The model under review builds one solid part; all positions refer to its coordinate system, in mm. A direction names the side the tool comes from. Coordinates: 2 decimals unless noted, no trailing zeros. Order: outer loops, then holes, each group sorted by start corner. A loop starts at its lowest first (then second) coordinate and runs counter-clockwise, first axis right, second up. Notation, with made-up numbers: M 35.5,67 L 50.5,67 A26 cw 50.5,91 Z; hole C 17.25,62.5 d10. An arc over 180 degrees is marked long. Answer in a Markdown table with one row per item.
from build123d import *

# Parameters (mm, degrees)
SKETCH_5_R                   = 50
EXTRUDE_1_DEPTH              = 35
SKETCH_2_W                   = 22
SKETCH_2_H                   = 20
CUT_EXTRUDE_1_DEPTH          = 165.975755795
HOLE_WIZARD_M6_1_D           = 6.6
HOLE_WIZARD_M6_1_CBORE_D     = 11
HOLE_WIZARD_M6_1_CBORE_DEPTH = 6.4
CUT_EXTRUDE_START            = -15
CUT_EXTRUDE_5_DEPTH          = 15
SKETCH_7_R                   = 5


with BuildPart() as part:
    # 草圖1 → 旋轉1 (revolve)
    with BuildSketch(Plane(origin=(0, 0, 0), x_dir=(0, 0, -1), z_dir=(1, 0, 0))):
        Polygon((0, 0), (0, 20), (50, 20), (114, 10), (114, 0), align=None)
    revolve(axis=Axis((0, 0, 0), (0, 1, 0)))

    # 草圖5 → 填料-伸長1 (add)
    with BuildSketch(Plane(origin=(0, 20, 0), x_dir=(1, 0, 0), z_dir=(0, 1, 0))):
        with Locations(Location((0, 0, 0), (0, 0, 270))):
            Circle(SKETCH_5_R)
    extrude(amount=-EXTRUDE_1_DEPTH)

    # 草圖2 → 除料-伸長1 (cut, through all)
    with BuildSketch(Plane(origin=(0, 20, 0), x_dir=(1, 0, 0), z_dir=(0, 1, 0))):
        with Locations((0, 18)):
            Rectangle(SKETCH_2_W, SKETCH_2_H)
    extrude(amount=-CUT_EXTRUDE_1_DEPTH, mode=Mode.SUBTRACT)

    # M6 六角承窩頭蓋螺釘的柱孔1 (through all)
    with Locations(Plane(origin=(0, 20, 0), x_dir=(1, 0, 0), z_dir=(0, 1, 0))):
        with Locations((37.5, 11), (22.5, 11), (-22.5, 11), (-37.5, 11)):
            CounterBoreHole(HOLE_WIZARD_M6_1_D / 2, HOLE_WIZARD_M6_1_CBORE_D / 2, HOLE_WIZARD_M6_1_CBORE_DEPTH)

    # 草圖6 → 除料-伸長5 (cut)
    with BuildSketch(Plane.XZ.offset(15).offset(CUT_EXTRUDE_START)):
        with BuildLine():
            Line((-37.563279942, 33), (37.563279942, 33))
            ThreePointArc((37.563279942, 33), (0, 50), (-37.563279942, 33))
        make_face()
        with BuildLine():
            ThreePointArc((-37.563279942, -33), (0, -50), (37.563279942, -33))
            Line((37.563279942, -33), (-37.563279942, -33))
        make_face()
    extrude(amount=CUT_EXTRUDE_5_DEPTH, mode=Mode.SUBTRACT)

    # 掃出1: sweep along a path in 草圖8
    with BuildLine(Plane.XY.offset(8)) as sweep_1_path:
        ThreePointArc((37.792366216, 20), (0, 57.792366216), (-37.792366216, 20))
    # 草圖7 → 掃出1 (sweep)
    with BuildSketch(Plane(origin=(0, 20, 0), x_dir=(1, 0, 0), z_dir=(0, 1, 0))):
        with Locations((38, -8)):
            Circle(SKETCH_7_R)
    sweep(path=sweep_1_path.line)


solid = part.part
(1) Take a section at B-B (x = 0). Write out the cut boundary in (y, z), then the cut area to 3 significant figures.
Report:
| item | result |
|---|---|
| outline | M -15,-33 L 0,-33 L 0,-114 L 10,-114 L 20,-50 L 20,-28 L -15,-28 Z; M -15,-8 L 20,-8 L 20,50 L 10,114 L 0,114 L 0,33 L -15,33 Z; C 58,8 d10 |
| area | 4,290 mm^2 |
(2) Take a section at A-A (y = 16.5). Write out the cut boundary in (x, z), then the cut area to 3 significant figures.
Report:
| item | result |
|---|---|
| outline | C 0,0 d144.8; hole C -37.5,-11 d11; hole C -22.5,-11 d11; hole M -11,-28 L 11,-28 L 11,-8 L -11,-8 Z; hole C 22.5,-11 d11; hole C 37.5,-11 d11 |
| area | 15,600 mm^2 |
(3) Take a section at C-C (z = -11). State how many separate pieces and enclosed holes the cut face has, then the cut area to 3 significant figures.
Report:
| item | result |
|---|---|
| separate pieces | 6 |
| enclosed holes | 0 |
| area | 3,550 mm^2 |
(4) Insertion check: P1, Ø8, axis at y = 1, z = 57, coming from the -X side; P2, Ø1.5, axis at x = -38.5, z = 50.5, coming from the +Y side; P3, Ø12, axis at y = -2, z = -23, coming from the -X side. Each pin has a flat end and moves straight along its axis. Give the tip position at first contact, or say it passes through.
Report:
| item | result |
|---|---|
| P1 | x = -100.93 |
| P2 | y = 18.01 |
| P3 | x = -112.67 |
(5) The part is to be moulded in two halves that separate along Z. For faces 1 (the flat face through (-34, 13.6, -11)), 2 (the cylindrical face through (43.66, 4.93, -105.31)), 3 (the flat face through (1, -15, 0)), say which applies: +Z half, -Z half, draft (parallel to the pull), parting line (faces both ways), or undercut.
Report:
| item | result |
|---|---|
| face 1 | undercut |
| face 2 | parting line |
| face 3 | draft |
(6) To check wall thickness, follow line 1 (X direction, y = 5.5, z = -11); line 2 (Y direction, x = -4, z = 17); line 3 (X direction, y = -1, z = -11) (3 decimals). State the ranges of each line that lie inside material, in increasing order. Write a range as [from, to].
Report:
| item | result |
|---|---|
| line 1 | [-113.47, -40.8], [-34.2, -25.8], [-19.2, -11], [11, 19.2], [25.8, 34.2], [40.8, 113.47] |
| line 2 | [-15, 20] |
| line 3 | [-48.775, -40.8], [-34.2, -25.8], [-19.2, -11], [11, 19.2], [25.8, 34.2], [40.8, 48.775] |
(7) Machinability: for faces 4 (the flat face through (11, 3, -18)), 5 (the flat face through (1, -7, -33)), 6 (the cylindrical face through (-49.997, -7.395, -0.505)), 7 (the cylindrical face through (49.997, -7.395, 0.505)), 8 (the cylindrical face through (-43, 17, -11)), which of the approach directions +Z, -Z, +X, -X, +Y, -Y give a long, thin tool a straight path to every point of the face, cutting with its end or side? Answer none if there is none.
Report:
| item | result |
|---|---|
| face 4 | +Y, -Y |
| face 5 | -Z, +X, -X, -Y |
| face 6 | -X, -Y |
| face 7 | +X, -Y |
| face 8 | +Y |
